Can you work these out from the model? Positions are in its coordinate system, mm. A direction names the side the tool comes from. Give positions to 0.01 mm unless a question says otherwise; leave off trailing zeros. Write each loop counter-clockwise with the first axis right and the second up, starting at its lowest first coordinate (ties: lowest second). Pieces come first, ordered by that corner, then holes. Notation, with made-up numbers: M 78,84 L 89,84 A24 ccw 89,118 Z; hole C -25.75,-10.5 d6. An arc over 180 degrees is marked long. Use CSV: the item, a comma, the result in double quotes. Start each with the question number.
from build123d import *

# Parameters (mm, degrees)
BASEHEAD_DEPTH = 2.8
BODYSKE_W      = 18.8
BODYSKE_H      = 2


with BuildPart() as part:
    # Sketch1 → BaseHead (new body)
    with BuildSketch(Plane(origin=(0, 0, 0), x_dir=(0, 0, -1), z_dir=(1, 0, 0))):
        Polygon((3.5, 2.020725942), (3.5, -2.020725942), (0, -4.041451884), (-3.5, -2.020725942), (-3.5, 2.020725942), (0, 4.041451884), align=None)
    extrude(amount=BASEHEAD_DEPTH)

    # BodySke → BaseBody (revolve)
    with BuildSketch(Plane.XY, mode=Mode.PRIVATE) as basebody_sk:
        with Locations((9.4, 1)):
            Rectangle(BODYSKE_W, BODYSKE_H)
    revolve(basebody_sk.sketch.rotate(Axis((0, 0, 0), (1, 0, 0)), 90), axis=Axis((0, 0, 0), (1, 0, 0)))

    # Sketch3 → HeadChamfer (revolve, cut)
    with BuildSketch(Plane.XY):
        Polygon((0, 3.5), (3.199358737, 9.041451884), (3.199358737, 14.041451884), (-10, 14.041451884), (-10, 3.5), align=None)
    revolve(axis=Axis((0, 0, 0), (1, 0, 0)), mode=Mode.SUBTRACT)


solid = part.part
(1) Which directions (+Z, -Z, +X, -X, +Y, -Y) give clear straight access to the entire face, cutting with the end or side of a thin tool? Please do faces 4 (the face through (1, 0, 3.5)), 5 (the face through (11, 2, 0)).
(2) Thinking about a two-plate mould opening in X: for faces 1 (the face through (18.8, 0, 0)), 2 (the face through (1.4, -3, -1.8)), 3 (the face through (0.076, -1.808, 3.149)), which applies, released by +X, released by -X, zero draft, split by the parting line, or undercut?
(3) Will these pins go through, and if not, where does the flat tip stop? pin 1 Ø1 at (y, z) = (-1.5, -2.5) entering from +X; pin 2 Ø3 at (x, z) = (3.5, 1) entering from +Y; pin 3 Ø1.5 at (x, y) = (15.5, 1.5) entering from +Z; pin 4 Ø3 at (x, z) = (12.5, 0.5) entering from +Y.
(4) Please list where these lines run through material, in increasing order: L1, parallel to X at y = 2.75, z = -1.25; L2, parallel to Y at x = 1, z = 1.75; L3, parallel to Z at x = 13, y = 0.25. Write a range as [from, to].
(5) I want a section at A-A (x = 8.75). Write out the boundary of the cut face in (y, z), and give its area (3 significant figures).
Geometry results:
1,face 4,"+Z, +X, -X, +Y, -Y"
1,face 5,"+X"
2,face 1,"released by +X"
2,face 2,"zero draft"
2,face 3,"released by -X"
3,pin 1,"stops at x = 2.8"
3,pin 2,"stops at y = 4.04"
3,pin 3,"stops at z = 1.85"
3,pin 4,"stops at y = 2"
4,L1,"x = [0, 2.8]"
4,L2,"y = [-3.03, 3.03]"
4,L3,"z = [-1.98, 1.98]"
5,outline,"C 0,0 d4"
5,area,"12.6 mm2"
